Source: CAD feature listing. Evaluate the final solid. Frame: model axes, mm. A direction names the side the tool comes from. Round coordinates to 2 decimals unless told otherwise and drop trailing zeros. Order: outer loops, then holes, each group sorted by start corner. A loop starts at its lowest first (then second) coordinate and runs counter-clockwise, first axis right, second up. Notation, with made-up numbers: (40, 73) -> (96, 73) arc R21 cw to (96, 80) -> close; hole circle Ø9 at (13, -4.75). An arc over 180 degrees is marked (long way). Use a Markdown table: item, result. Add a question column.
```python
from build123d import *

# Parameters (mm, degrees)
F0_W      = 40
F0_H      = 25
F1_DEPTH  = 10
F2_W      = 6
F2_H      = 25
F3_DEPTH  = 6
F4_R      = 2.99999
F5_R      = 1
F6_DEPTH  = 30
F7_SIZE   = 6
F8_R      = 1
F9_DEPTH  = 1
F10_R     = 1
F11_DEPTH = 1


# Not quite as in the source:
# - a fillet or chamfer is up to 0.001 mm smaller than in the source, because OpenCascade refuses the exact size
# - ends of sketch curves that miss each other by under 0.0002 mm in the source are joined


with BuildPart() as f1:
    # F0 (on Top) → F1 (new body)
    with BuildSketch(Plane.XY):
        Rectangle(F0_W, F0_H)
    extrude(amount=F1_DEPTH)

    # F2 (on face) → F3 (join)
    with BuildSketch(Plane(origin=(0, 0, 0), x_dir=(1, 0, 0), z_dir=(0, 0, -1))):
        with Locations((9, 0)):
            Rectangle(F2_W, F2_H)
    extrude(amount=F3_DEPTH)

    # F4 (radius 3 in the source; OpenCascade refuses exactly that, so slightly less here)
    f4_edges = [f1.edges().sort_by_distance(p)[0] for p in [
        (6, 0, -6),
        (12, 0, -6),
    ]]
    fillet(f4_edges, radius=F4_R)

    # F5 (on face) → F6 (cut)
    with BuildSketch(Plane(origin=(0, 12.5, 0), x_dir=(-1, 0, 0), z_dir=(0, 1, 0))):
        with Locations((-9, -3)):
            Circle(F5_R)
    extrude(amount=-F6_DEPTH, mode=Mode.SUBTRACT)

    # F7
    f7_edges = [f1.edges().sort_by_distance(p)[0] for p in [
        (20, 0, 0),
    ]]
    chamfer(f7_edges, length=F7_SIZE)

    # F8 (on face) → F9 (cut)
    with BuildSketch(Plane(origin=(0, 12.5, 0), x_dir=(-1, 0, 0), z_dir=(0, 1, 0))):
        with BuildLine():
            Line((-6, -3.00001), (-6, 0))
            Line((-6, 0), (-12, 0))
            Line((-12, 0), (-12, -3.00001))
            ThreePointArc((-12, -3.00001), (-11.1213232725, -5.1213232725), (-9.00001, -6))
            ThreePointArc((-9.00001, -6), (-6.8786767275, -5.1213232725), (-6, -3.00001))
        make_face()
        with Locations((-9, -3)):
            Circle(F8_R, mode=Mode.SUBTRACT)
    extrude(amount=-F9_DEPTH, mode=Mode.SUBTRACT)

    # F10 (on face) → F11 (cut)
    with BuildSketch(Plane.XZ.offset(12.5)):
        with BuildLine():
            Line((12, 0), (6, 0))
            Line((6, 0), (6, -3.00001))
            ThreePointArc((6, -3.00001), (6.8786767275, -5.1213232725), (8.99999, -6))
            ThreePointArc((8.99999, -6), (11.1213232725, -5.1213232725), (12, -3.00001))
            Line((12, -3.00001), (12, 0))
        make_face()
        with Locations((9, -3)):
            Circle(F10_R, mode=Mode.SUBTRACT)
    extrude(amount=-F11_DEPTH, mode=Mode.SUBTRACT)


solid = f1.part
```
1) Line query: probe 1 along Z at (x, y) = (4.5, -3); probe 2 along X at (y, z) = (10, -3.25); probe 3 along X at (y, z) = (-0.25, -3.75). Output: solid intervals per line, ascending. Write a range as from..to.
2) Draft query along Z for faces 1 (the cylindrical face through (9.8, 0.2, -3.6)), 2 (the flat face through (20, 0, 8)), 3 (the cylindrical face through (6.86, -0.16, -5.1)). Return one class per face: pulls with the +Z half, pulls with the -Z half, needs draft (parallel to the pull), parting line crosses it, or undercut.
3) Section C-C on x = -3.5. Output: boundary loops of the cut face in (y, z).
4) First-contact query: pin 1 Ø1.8 at (x, z) = (10, -3.5) entering from +Y; pin 2 Ø0.9 at (y, z) = (-0.5, -1) entering from -X; pin 3 Ø4 at (y, z) = (8, 3) entering from +X. Flat tips, straight axial feed; report the tip coordinate or a pass-through.
5) Reachability of faces 4 (the flat face through (8, -11.5, -2)), 5 (the flat face through (-20, 0, 5)), 6 (the flat face through (6, 0, -1)), 7 (the flat face through (12, 0, -1)), 8 (the flat face through (10, 11.5, -2)) from +Z, -Z, +X, -X, +Y, -Y: full face, straight path, thin tool, end or side. Return the list, or none.
6) Section B-B on z = 1.25. Output: boundary loops of the cut face in (x, y), then the cut area to 3 significant figures.
Conclusion:
| question | item | result |
|---|---|---|
| 1 | probe 1 | z = 0..10 |
| 1 | probe 2 | x = 6.01..8.03, 9.97..11.99 |
| 1 | probe 3 | x = 6.1..8.34, 9.66..11.9 |
| 2 | face 1 | undercut |
| 2 | face 2 | needs draft |
| 2 | face 3 | pulls with the -Z half |
| 3 | outline | (-12.5, 0) -> (12.5, 0) -> (12.5, 10) -> (-12.5, 10) -> close |
| 4 | pin 1 | stops at y = 11.5 |
| 4 | pin 2 | stops at x = 6 |
| 4 | pin 3 | stops at x = 19 |
| 5 | face 4 | -Z, +X, -X, -Y |
| 5 | face 5 | +Z, -Z, -X, +Y, -Y |
| 5 | face 6 | -Z, -X, +Y, -Y |
| 5 | face 7 | -Z, +X, +Y, -Y |
| 5 | face 8 | -Z, +X, -X, +Y |
| 6 | outline | (-20, -12.5) -> (15.25, -12.5) -> (15.25, 12.5) -> (-20, 12.5) -> close |
| 6 | area | 881 mm^2 |
